Verification items for the finished model (mm, model axes). A direction names the side the tool comes from. Give positions to 0.01 mm unless a question says otherwise; leave off trailing zeros. Order: outer loops, then holes, each group sorted by start corner. A loop starts at its lowest first (then second) coordinate and runs counter-clockwise, first axis right, second up. Notation, with made-up numbers: (15, -4) - (46, -4) arc R31 ccw to (46, 23) - close; hole circle Ø10 at (38, 54). An arc over 180 degrees is marked (long way). Answer as a JSON object with one key per item and string values. Group by question number.
(1) Section check D-D (z = -155.5). Record the boundary of the cut face in (x, y).
(2) Depth check by flat-ended pin: pin 1 Ø1 at (y, z) = (105, -32) entering from -X; pin 2 Ø12 at (x, y) = (-134, 78) entering from +Z; pin 3 Ø10 at (x, y) = (-28, 50) entering from -Z. Enter the tip coordinate at first touch or a pass-through.
(3) Section check B-B (x = -100). Record the boundary of the cut face in (y, z), then the cut area to 3 significant figures.
(4) Section check C-C (y = 142). Record the boundary of the cut face in (x, z), then the cut area to 3 significant figures.
(5) Access from +Z, -Z, +X, -X, +Y, -Y to the whole of each face (thin tool, end or side, straight path). Record for faces 1 (the face through (-140, 205, -130)), 2 (the face through (-99, 99, -11.709)), 3 (the face through (-190, 99, -99)).
(6) Thickness scan on line 1 (Y direction, x = -80.5, z = -9); line 2 (Z direction, x = -100, y = 171); line 3 (X direction, y = 184, z = -100). Record the ranges inside material, lowest first.
(7) Section check A-A (z = -100). Record the boundary of the cut face in (x, y).
(8) Mould release check, pull along X, two halves, no side actions. Record for faces 4 (the face through (-99, 170, -200)), 5 (the face through (0, 170, -99)), 6 (the face through (-61.847, 190.56, -112.015)): +X half, -X half, draft (parallel to the pull), parting line (faces both ways), or undercut.
Autodesk Inventor part; units mm, degrees
ref_plane "YZ Plane" through (0, 0, 0) normal (1, 0, 0) x (0, 1, 0)
ref_plane "XZ Plane" through (0, 0, 0) normal (0, 1, 0) x (-1, 0, 0)
ref_plane "XY Plane" through (0, 0, 0) normal (0, 0, 1) x (1, 0, 0)
sketch "Sketch1" plane through (0, 0, 0) normal (0, 1, 0) x (-1, 0, 0)
  line L0 (0, 0) -> (200, 0)
  line L1 (200, 0) -> (200, -200)
  line L2 (200, -200) -> (0, -200)
  line L3 (0, -200) -> (0, 0)
  dimension "d0" = 200
  dimension "d1" = 200
extrude "Extrusion1" add sketch "Sketch1" along normal blind 40
sketch "Sketch2" plane through (0, 40, 0) normal (0, 1, 0) x (1, 0, 0)
  line L0 (0, 200) -> (-200, 200)
  line L1 (-200, 200) -> (-200, 0)
  line L2 (-200, 0) -> (0, 0)
  line L3 (0, 0) -> (0, 200)
  line L4 (-10, 11.7093) -> (-190, 11.7093)
  line L5 (-190, 11.7093) -> (-190, 188.2907)
  line L6 (-190, 188.2907) -> (-10, 188.2907)
  line L7 (-10, 188.2907) -> (-10, 11.7093)
  line L8 (-10, 11.7093) -> (-190, 188.2907) construction
  line L9 (-190, 11.7093) -> (-10, 188.2907) construction
  point P0 (-100, 100)
  dimension "d4" = 180
extrude "Extrusion2" add sketch "Sketch2" along normal blind 120 contours L4 L5 L6 L7
sketch "Sketch3" plane through (0, 160, 0) normal (0, 1, 0) x (1, 0, 0)
  line L0 (-10, 188.2907) -> (-190, 188.2907)
  line L1 (-190, 188.2907) -> (-190, 11.7093)
  line L2 (-190, 11.7093) -> (-10, 11.7093)
  line L3 (-10, 11.7093) -> (-10, 188.2907)
  line L4 (0, 0) -> (0, 200)
  line L5 (0, 200) -> (-200, 200)
  line L6 (0, 0) -> (-200, 0)
  line L7 (-200, 0) -> (-200, 200)
  line L8 (-200, 200) -> (0, 200)
  line L9 (0, 200) -> (0, 0)
extrude "Extrusion3" add sketch "Sketch3" along normal blind 20 contours L3 L2 L1 L0 | L6 L7 L5 L4
sketch "Sketch4" plane through (0, 180, 0) normal (0, 1, 0) x (1, 0, 0)
  line L0 (-200, 200) -> (-200, 0)
  line L1 (-200, 200) -> (0, 0)
  line L2 (0, 200) -> (-200, 200)
  line L3 (-200, 0) -> (0, 200)
  circle A0 centre (-100, 100) radius 50
  dimension "d9" = 100
extrude "Extrusion4" add sketch "Sketch4" along normal blind 50 contours A0 L3 L1 | L1 L3 A0 | L3 L1 A0 | L3 A0 L1
sketch "Sketch5" plane through (-100, 230, -100) normal (0, 1, 0) x (1, 0, 0)
  circle A0 centre (0, 0) radius 40
  point P0 (100, -100)
  dimension "d12" = 80
extrude "Extrusion5" cut sketch "Sketch5" against normal blind 80
properties part number "Camara"
Solutions:
{
 "1": {"outline": "(-200, 0) - (0, 0) - (0, 40) - (-10, 40) - (-10, 160) - (0, 160) - (0, 180) - (-200, 180) - (-200, 160) - (-190, 160) - (-190, 40) - (-200, 40) - close"},
 "2": {"pin 1": "stops at x = -190", "pin 2": "stops at z = -11.71", "pin 3": "stops at z = -188.29"},
 "3": {"outline": "(0, -200) - (40, -200) - (40, -188.29) - (160, -188.29) - (160, -200) - (180, -200) - (180, -150) - (230, -150) - (230, -140) - (150, -140) - (150, -60) - (230, -60) - (230, -50) - (180, -50) - (180, 0) - (160, 0) - (160, -11.71) - (40, -11.71) - (40, 0) - (0, 0) - close", "area": "31,800 mm2"},
 "4": {"outline": "(-190, -188.29) - (-10, -188.29) - (-10, -11.71) - (-190, -11.71) - close", "area": "31,800 mm2"},
 "5": {"face 1": "+Y", "face 2": "+Z, +X, -X", "face 3": "+Z, -Z, -X"},
 "6": {"line 1": "y = 0 to 40, 160 to 180", "line 2": "z = -200 to -140, -60 to 0", "line 3": "x = -150 to -140, -60 to -50"},
 "7": {"outline": "(-200, 0) - (0, 0) - (0, 40) - (-10, 40) - (-10, 160) - (0, 160) - (0, 180) - (-50, 180) - (-50, 230) - (-60, 230) - (-60, 150) - (-140, 150) - (-140, 230) - (-150, 230) - (-150, 180) - (-200, 180) - (-200, 160) - (-190, 160) - (-190, 40) - (-200, 40) - close"},
 "8": {"face 4": "draft", "face 5": "+X half", "face 6": "undercut"}
}
